Source: CAD feature listing. Evaluate the final solid. Frame: model axes, mm. A direction names the side the tool comes from. Give positions to 0.01 mm unless a question says otherwise; leave off trailing zeros. Write each loop counter-clockwise with the first axis right and the second up, starting at its lowest first coordinate (ties: lowest second). Pieces come first, ordered by that corner, then holes. Notation, with made-up numbers: (25.5, 26.5) -> (36.5, 26.5) arc R19 cw to (36.5, 61.5) -> close; hole circle Ø6 at (-26.5, 53). An arc over 180 degrees is marked (long way). Use a Markdown table: item, result. Add a question column.
```python
from build123d import *

# Parameters (mm, degrees)
SKETCH_1_W          = 12
SKETCH_1_H          = 6
EXTRUDE_1_DEPTH     = 14
SKETCH_2_R          = 2.5
CUT_EXTRUDE_1_DEPTH = 14
SKETCH_4_R          = 1.5
CUT_EXTRUDE_2_DEPTH = 28
SKETCH_5_R          = 5.5
CUT_EXTRUDE_3_DEPTH = 22


with BuildPart() as part:
    # 草图1 → 凸台-拉伸1 (new body)
    with BuildSketch(Plane.XY):
        with BuildLine():
            Line((-2.226515598, 16.75), (-11.726515598, 16.75))
            Line((-11.726515598, 16.75), (-11.726515598, -10.25))
            Line((-11.726515598, -10.25), (-11.726515598, -16.25))
            Line((-11.726515598, -16.25), (10.273484402, -16.25))
            Line((10.273484402, -16.25), (10.273484402, -10.25))
            Line((10.273484402, -10.25), (10.273484402, 16.75))
            Line((10.273484402, 16.75), (0.773484402, 16.75))
            Line((0.773484402, 16.75), (0.773484402, 9.992640687))
            ThreePointArc((0.773484402, 9.992640687), (2.947719016, 8.348076211), (3.773484402, 5.75))
            ThreePointArc((3.773484402, 5.75), (-3.324591809, 2.075765386), (-2.226515598, 9.992640687))
            Line((-2.226515598, 9.992640687), (-2.226515598, 16.75))
        make_face()
        with Locations((16.273484402, -13.25)):
            Rectangle(SKETCH_1_W, SKETCH_1_H)
        with Locations((-17.726515598, -13.25)):
            Rectangle(SKETCH_1_W, SKETCH_1_H)
    extrude(amount=EXTRUDE_1_DEPTH)

    # 草图2 → 切除-拉伸1 (cut)
    with BuildSketch(Plane(origin=(0, -16.25, 0), x_dir=(-1, 0, 0), z_dir=(0, -1, 0))):
        with Locations(Location((18.726515598, -7, 0), (0, 0, 180))):
            Circle(SKETCH_2_R)
        with Locations(Location((-17.273484402, -7, 0), (0, 0, 270))):
            Circle(SKETCH_2_R)
    extrude(amount=-CUT_EXTRUDE_1_DEPTH, mode=Mode.SUBTRACT)

    # 草图4 → 切除-拉伸2 (cut)
    with BuildSketch(Plane.ZY.offset(11.726515598)):
        with Locations(Location((7, 13.75, 0), (0, 0, 90))):
            Circle(SKETCH_4_R)
    extrude(amount=-CUT_EXTRUDE_2_DEPTH, mode=Mode.SUBTRACT)

    # 草图5 → 切除-拉伸3 (cut)
    with BuildSketch(Plane.XY.offset(14)):
        with Locations((-0.726515598, 5.75)):
            Circle(SKETCH_5_R)
    extrude(amount=-CUT_EXTRUDE_3_DEPTH, mode=Mode.SUBTRACT)


solid = part.part
```
(1) Cut plane B-B on z = 7. Return the cut outline in (x, y), then the cut area to 3 significant figures.
(2) Cut plane D-D on x = -9. Return the cut outline in (y, z).
(3) First-contact query: pin 1 Ø4 at (y, z) = (13.75, 7) entering from -X; pin 2 Ø1.7 at (y, z) = (13, 8) entering from +X; pin 3 Ø6 at (x, z) = (17.5, 8) entering from +Y; pin 4 Ø2.5 at (y, z) = (13.75, 7) entering from -X. Flat tips, straight axial feed; report the tip coordinate or a pass-through.
(4) Cut plane C-C on y = 14. Return the cut outline in (x, z), then the cut area to 3 significant figures.
(5) Mould query, pull axis Z, two halves, no side actions, for faces 4 (the flat face through (-1, -3, 0)), 5 (the cylindrical face through (-0.947, 0.254, 7.098)), 6 (the cylindrical face through (-16.42, -13.29, 6.04)). Classes: +Z half, -Z half, draft (parallel to the pull), parting line (faces both ways), or undercut.
(6) Cut plane A-A on y = 5.75. Return the cut outline in (x, z).
(7) Material intervals for L1, parallel to Y at x = -6.5, z = 7; L2, parallel to Z at x = 6.75, y = 13.75; L3, parallel to X at y = 15.5, z = 5.75, sorted ascending.
(8) Access query for faces 1 (the flat face through (14.9, -10.25, 8.5)), 2 (the flat face through (-16, -10.25, 5)), 3 (the flat face through (-2.227, 14, 5)). Directions: +Z, -Z, +X, -X, +Y, -Y. A direction counts if a zero-diameter tool reaches every point of the face in a straight line with its end or side. Return the directions, or none.
Output:
| question | item | result |
|---|---|---|
| 1 | outline | (-23.73, -16.25) -> (-21.23, -16.25) -> (-21.23, -10.25) -> (-23.73, -10.25) -> close; (-16.23, -16.25) -> (14.77, -16.25) -> (14.77, -10.25) -> (10.27, -10.25) -> (10.27, 12.25) -> (0.77, 12.25) -> (0.77, 11.04) arc R5.5 cw (long way) to (-2.23, 11.04) -> (-2.23, 12.25) -> (-11.73, 12.25) -> (-11.73, -10.25) -> (-16.23, -10.25) -> close; (-11.73, 15.25) -> (-2.23, 15.25) -> (-2.23, 16.75) -> (-11.73, 16.75) -> close; (0.77, 15.25) -> (10.27, 15.25) -> (10.27, 16.75) -> (0.77, 16.75) -> close; (19.77, -16.25) -> (22.27, -16.25) -> (22.27, -10.25) -> (19.77, -10.25) -> close |
| 1 | area | 641 mm^2 |
| 2 | outline | (-16.25, 0) -> (16.75, 0) -> (16.75, 14) -> (-16.25, 14) -> close; hole circle Ø3 at (13.75, 7) |
| 3 | pin 1 | x = -11.73 |
| 3 | pin 2 | x = 10.27 |
| 3 | pin 3 | y = -10.25 |
| 3 | pin 4 | through |
| 4 | outline | (-11.73, 0) -> (-2.23, 0) -> (-2.23, 5.52) -> (-11.73, 5.52) -> close; (-11.73, 8.48) -> (-2.23, 8.48) -> (-2.23, 14) -> (-11.73, 14) -> close; (0.77, 0) -> (10.27, 0) -> (10.27, 5.52) -> (0.77, 5.52) -> close; (0.77, 8.48) -> (10.27, 8.48) -> (10.27, 14) -> (0.77, 14) -> close |
| 4 | area | 210 mm^2 |
| 5 | face 4 | -Z half |
| 5 | face 5 | draft |
| 5 | face 6 | undercut |
| 6 | outline | (-11.73, 0) -> (-6.23, 0) -> (-6.23, 14) -> (-11.73, 14) -> close; (4.77, 0) -> (10.27, 0) -> (10.27, 14) -> (4.77, 14) -> close |
| 7 | L1 | -16.25 to 12.25, 15.25 to 16.75 |
| 7 | L2 | 0 to 5.5, 8.5 to 14 |
| 7 | L3 | -11.73 to -2.23, 0.77 to 10.27 |
| 8 | face 1 | +Z, -Z, +X, +Y |
| 8 | face 2 | +Z, -Z, -X, +Y |
| 8 | face 3 | +Z, -Z, +Y |
